Build history of the part. All positions in model axes, mm. A direction names the side the tool comes from. Give positions to 0.01 mm unless a question says otherwise; leave off trailing zeros. Loops run counter-clockwise (first coordinate to the right, second up) from the corner with the lowest first, then second, coordinate; pieces in that order, holes last.
1) Flat gauge pins, fed straight in: P1, Ø8, axis at x = 5.5, z = 5.5, coming from the -Y side; P2, Ø2, axis at x = 11, y = 4.5, coming from the +Z side; P3, Ø3, axis at y = 4.5, z = -6.5, coming from the -X side; P4, Ø2, axis at y = 8.5, z = 3, coming from the -X side. Where does each tip first touch, or does it go through?
2) Band-saw the part on B-B on x = 0. List the corners of the cut face in (y, z).
3) Band-saw the part on A-A on y = 11.25. List the corners of the cut face in (x, z).
4) Wall check: line 1 (Z direction, x = 0, y = 10.7); line 2 (Z direction, x = 0, y = 2); line 3 (X direction, y = 11.1, z = 0). Give the ranges that are in metal, low to high.
5) 3-axis set-ups, long thin cutter, end or side, ignore diameter. For faces 5 (the flat face through (2, 9.652, -10)), 6 (the cylindrical face through (-10.45, 5.92, -21.04)): which of +Z, -Z, +X, -X, +Y, -Y reach the whole face in a straight line?
6) Band-saw the part on C-C on y = 9. List the corners of the cut face in (x, z), then the cut area to 3 significant figures.
7) Two-plate mould, pull along Z, no slides. Class faces 1 (the flat face through (0, 0, -12)), 2 (the flat face through (13.1, 5.76, -11.52)), 3 (the cylindrical face through (12.2, 10.94, 5.06)), 4 (the cylindrical face through (5.36, 4.894, -8.406)): +Z half, -Z half, draft (parallel to the pull), parting line (faces both ways), or undercut.
```python
from build123d import *

# Parameters (mm, degrees)
EXTRUDE1_DEPTH = 12.192
FILLET2_R      = 2.54
FILLET1_R      = 0.508
SKETCH6_R      = 9.9695
EXTRUDE2_DEPTH = 13.192
SKETCH7_R      = 13.208
EXTRUDE3_DEPTH = 2.54


with BuildPart() as part:
    # Sketch5 → Extrude1 (new body)
    with BuildSketch(Plane(origin=(0, 0, 0), x_dir=(1, 0, 0), z_dir=(0, 1, 0))):
        with BuildLine():
            Line((-10.922, 21.59), (10.922, 21.59))
            Line((10.922, 21.59), (14.895447762, 3.222302897))
            ThreePointArc((14.895447762, 3.222302897), (0, -15.24), (-14.895447762, 3.222302897))
            Line((-14.895447762, 3.222302897), (-10.922, 21.59))
        make_face()
    extrude(amount=EXTRUDE1_DEPTH)

    # Fillet2
    fillet2_edges = [part.edges().sort_by_distance(p)[0] for p in [
        (-10.922, 6.096, -21.59),
        (10.922, 6.096, -21.59),
    ]]
    fillet(fillet2_edges, radius=FILLET2_R)

    # Fillet1
    fillet1_edges = [part.edges().sort_by_distance(p)[0] for p in [
        (13.125370945, 12.192, -11.40467669),
        (-13.125370945, 12.192, -11.40467669),
        (0, 12.192, -21.59),
        (10.467632001, 12.192, -21.026829308),
        (-10.467632001, 12.192, -21.026829308),
        (0, 12.192, 15.24),
    ]]
    fillet(fillet1_edges, radius=FILLET1_R)

    # Sketch6 → Extrude2 (cut, through all)
    with BuildSketch(Plane(origin=(0, 12.192, 0), x_dir=(1, 0, 0), z_dir=(0, 1, 0))):
        Circle(SKETCH6_R)
    extrude(amount=-EXTRUDE2_DEPTH, mode=Mode.SUBTRACT)

    # Sketch7 → Extrude3 (cut)
    with BuildSketch(Plane(origin=(0, 12.192, 0), x_dir=(1, 0, 0), z_dir=(0, 1, 0))):
        Circle(SKETCH7_R)
    extrude(amount=-EXTRUDE3_DEPTH, mode=Mode.SUBTRACT)


solid = part.part
```
Findings below:
1. P1: stops at y = 0
1. P2: stops at z = 11.5
1. P3: stops at x = -14.51
1. P4: stops at x = -15.11
2. outline: (0, -21.59) - (11.68, -21.59) arc R0.51 ccw to (12.19, -21.08) - (12.19, -13.21) - (9.65, -13.21) - (9.65, -9.97) - (0, -9.97) - close; (0, 9.97) - (9.65, 9.97) - (9.65, 13.21) - (12.19, 13.21) - (12.19, 14.73) arc R0.51 ccw to (11.68, 15.24) - (0, 15.24) - close
3. outline: (-14.9, -3.22) - (-11.36, -19.59) arc R2.54 ccw to (-8.87, -21.59) - (8.87, -21.59) arc R2.54 ccw to (11.36, -19.59) - (14.9, -3.22) arc R15.24 ccw (long way) to start; hole circle Ø26.42 at (0, 0)
4. line 1: z = -21.59 to -13.21, 13.21 to 15.24
4. line 2: z = -21.59 to -9.97, 9.97 to 15.24
4. line 3: x = -15.24 to -13.21, 13.21 to 15.24
5. face 5: +Y
5. face 6: -Z, -X, +Y, -Y
6. outline: (-14.9, -3.22) - (-11.36, -19.59) arc R2.54 ccw to (-8.87, -21.59) - (8.87, -21.59) arc R2.54 ccw to (11.36, -19.59) - (14.9, -3.22) arc R15.24 ccw (long way) to start; hole circle Ø19.94 at (0, 0)
6. area: 623 mm2
7. face 1: draft
7. face 2: -Z half
7. face 3: undercut
7. face 4: undercut
